Could you check a few things on this model? Use its own coordinates, in mm. Round coordinates to 2 decimals unless told otherwise and drop trailing zeros. Loops run counter-clockwise (first coordinate to the right, second up) from the corner with the lowest first, then second, coordinate; pieces in that order, holes last. Notation, with made-up numbers: M 55,40.25 L 102,40.25 A11 ccw 102,58.25 Z; hole C 27,14.25 d9. An arc over 180 degrees is marked long. One line per item, written item: value. Start each with the question number.
Q1. Imagine slicing it at C-C (y = 99.5). Please give me the cut outline in (x, z), then the cut area to 3 significant figures.
Q2. Imagine slicing it at A-A (x = 10.5). Please give me the cut outline in (y, z).
Q3. Imagine slicing it at B-B (z = -442). Please give me the cut outline in (x, y), then the cut area to 3 significant figures.
Q4. I'm going to push flat-ended pins straight in: pin 1 Ø4 at (x, y) = (6.5, 48) entering from +Z; pin 2 Ø3 at (y, z) = (24.5, -91) entering from +X; pin 3 Ø3 at (y, z) = (148.7, -506.62) entering from +X; pin 4 Ø3 at (y, z) = (23, -91) entering from -X. Where does each tip first touch, or does it pass through?
Q5. Please list where these lines run through material, in increasing order: line 1 along Y through (x, z) = (3.5, -97.5); line 2 along Y through (x, z) = (5.5, -181); line 3 along Y through (x, z) = (5.5, -491).
from build123d import *

# Parameters (mm, degrees)
BOSS_EXTRUDE1_DEPTH = 12.7
FILLET1_R           = 76.2
FILLET2_R           = 50.8
FILLET3_R           = 12.7
SKETCH1_3_R         = 1.778
CUT_EXTRUDE1_DEPTH  = 32.004
SKETCH1_5_R         = 1.778
CUT_EXTRUDE3_DEPTH  = 19.304
SKETCH2_W           = 20
SKETCH2_H           = 5
CUT_EXTRUDE4_DEPTH  = 5
CUT_EXTRUDE5_DEPTH  = 5


with BuildPart() as part:
    # Sketch1 → Boss-Extrude1 (new body)
    with BuildSketch(Plane(origin=(0, 0, 0), x_dir=(0, 0, -1), z_dir=(1, 0, 0))):
        Polygon((-60.216908745, 47.566393508), (-60.216908745, -26.034482759), (-31.989836752, -26.034482759), (536.590579473, 7.973019947), (536.590579473, 211.173019947), align=None)
    extrude(amount=BOSS_EXTRUDE1_DEPTH)

    # Fillet1
    fillet1_edges = [part.edges().sort_by_distance(p)[0] for p in [
        (6.35, 47.566393508, 60.216908745),
    ]]
    fillet(fillet1_edges, radius=FILLET1_R)

    # Fillet2
    fillet2_edges = [part.edges().sort_by_distance(p)[0] for p in [
        (6.35, 211.173019947, -536.590579473),
    ]]
    fillet(fillet2_edges, radius=FILLET2_R)

    # Fillet3
    fillet3_edges = [part.edges().sort_by_distance(p)[0] for p in [
        (6.35, -26.034482759, 60.216908745),
    ]]
    fillet(fillet3_edges, radius=FILLET3_R)

    # Sketch1<3> → Cut-Extrude1 (cut)
    with BuildSketch(Plane(origin=(0, 0, 0), x_dir=(0, 0, -1), z_dir=(1, 0, 0))):
        with Locations((503.316579473, 54.583559733)):
            Circle(SKETCH1_3_R)
    extrude(amount=CUT_EXTRUDE1_DEPTH, mode=Mode.SUBTRACT)

    # Sketch1<5> → Cut-Extrude3 (cut)
    with BuildSketch(Plane(origin=(0, 0, 0), x_dir=(0, 0, -1), z_dir=(1, 0, 0))):
        with Locations((506.618579473, 148.702123969)):
            Circle(SKETCH1_5_R)
    extrude(amount=CUT_EXTRUDE3_DEPTH, mode=Mode.SUBTRACT)

    # Sketch2 → Cut-Extrude4 (cut)
    with BuildSketch(Plane(origin=(12.7, -3.610856195, -1.673147661), x_dir=(0, 0.05233595624294395, -0.9986295347545739), z_dir=(1, 0, 0))):
        with Locations((94.879123185, 22.820976731)):
            Rectangle(SKETCH2_W, SKETCH2_H)
    extrude(amount=-CUT_EXTRUDE4_DEPTH, mode=Mode.SUBTRACT)

    # Sketch3 → Cut-Extrude5 (cut)
    with BuildSketch(Plane.ZY):
        Polygon((-85.110749427, 26.117649094), (-85.372429208, 21.12450142), (-105.345019904, 22.171220545), (-105.083340122, 27.164368219), align=None)
    extrude(amount=-CUT_EXTRUDE5_DEPTH, mode=Mode.SUBTRACT)


solid = part.part
Report:
1. outline: M 0,-536.59 L 12.7,-536.59 L 12.7,-129.23 L 0,-129.23 Z
1. area: 5,170 mm²
2. outline: M -26.03,31.99 L 7.97,-536.59 L 144.57,-536.59 A50.8 ccw 193.57,-472.36 L 62.93,4.16 A76.2 ccw -10.56,60.22 L -13.33,60.22 A12.7 ccw -26.03,47.52 Z; hole M 21.12,-85.37 L 22.17,-105.35 L 27.16,-105.08 L 26.12,-85.11 Z; hole C 54.58,-503.32 d3.56; hole C 148.7,-506.62 d3.56
3. outline: M 0,2.32 L 12.7,2.32 L 12.7,185.24 L 0,185.24 Z
3. area: 2,320 mm²
4. pin 1: stops at z = 35.08
4. pin 2: stops at x = 7.7
4. pin 3: passes through
4. pin 4: stops at x = 5
5. line 1: y = -18.29 to 21.76, 26.77 to 90.8
5. line 2: y = -13.3 to 113.69
5. line 3: y = 5.25 to 195.1
